Source: three-view drawing plus pictorial views. Frame: mm from the lowest corner of the part. Give positions to 0.01 mm unless a question says otherwise; leave off trailing zeros. Loops run counter-clockwise (first coordinate to the right, second up) from the corner with the lowest first, then second, coordinate; pieces in that order, holes last. Notation, with made-up numbers: (-36.75, 2) -> (-1.75, 2) arc R18 cw to (-1.75, 27) -> close; hole circle Ø3 at (54, 44.5). An arc over 180 degrees is marked (long way). Put each result on its own line as item: value.
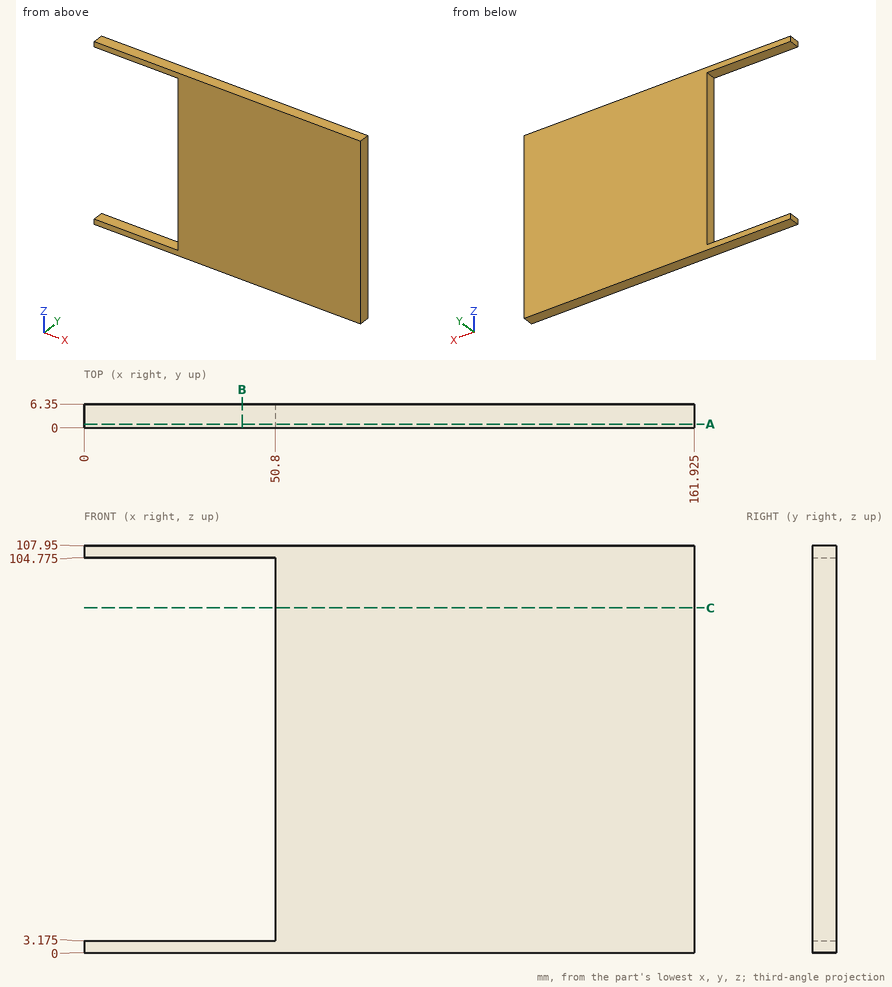
(1) First-contact query: P1, Ø3, axis at y = 2, z = 83, coming from the -X side. Flat tip, straight axial feed; report the tip coordinate or a pass-through.
Calculated:
P1: stops at x = 50.8
(2) Section C-C on z = 91.5. Return loops of the section in (x, y) (3 decimals).
Calculated:
outline: (50.8, 0) -> (161.925, 0) -> (161.925, 6.35) -> (50.8, 6.35) -> close
(3) Section B-B on x = 42. Return loops of the section in (y, z) (3 decimals).
Calculated:
outline: (0, 0) -> (6.35, 0) -> (6.35, 3.175) -> (0, 3.175) -> close; (0, 104.775) -> (6.35, 104.775) -> (6.35, 107.95) -> (0, 107.95) -> close
(4) Line query: probe 1 along Z at (x, y) = (18, 3) (3 decimals); probe 2 along X at (y, z) = (5.5, 27) (3 decimals). Output: solid intervals per line, ascending. Write a range as from..to.
Calculated:
probe 1: z = 0..3.175, 104.775..107.95
probe 2: x = 50.8..161.925
(5) Section A-A on y = 1. Return loops of the section in (x, z) (3 decimals).
Calculated:
outline: (0, 0) -> (161.925, 0) -> (161.925, 107.95) -> (0, 107.95) -> (0, 104.775) -> (50.8, 104.775) -> (50.8, 3.175) -> (0, 3.175) -> close
